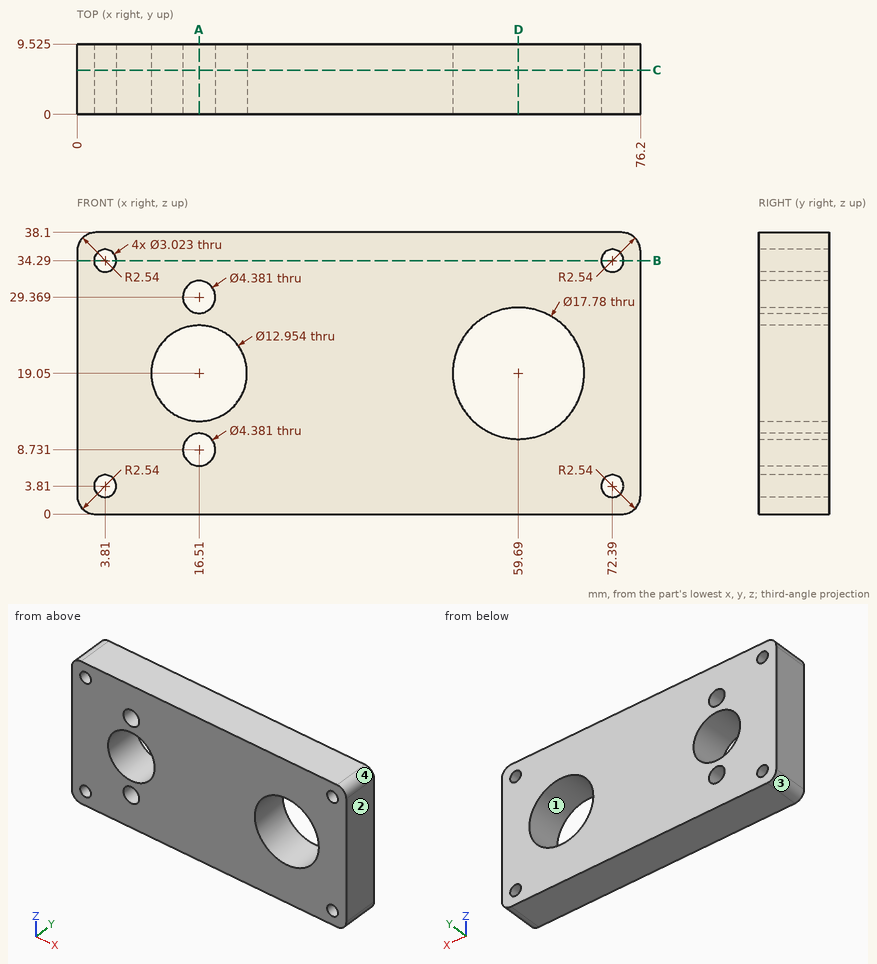
Verification items for this drawing (mm, ordinates from the low corner). Coordinates: 2 decimals unless noted, no trailing zeros. Loops run counter-clockwise (first coordinate to the right, second up) from the corner with the lowest first, then second, coordinate; pieces in that order, holes last. Notation, with made-up numbers: (-33, 28.5) -> (-26, 28.5) arc R18 cw to (-26, 62.5) -> close; hole circle Ø1 at (-21, 62). An arc over 180 degrees is marked (long way). Put each result on its own line as item: value.
1. Section check A-A, the plane x = 16.51. Record the boundary of the cut face in (y, z) (1 decimal), then the cut area to 3 significant figures.
Result set:
outline: (0, 0) -> (9.5, 0) -> (9.5, 6.5) -> (0, 6.5) -> close; (0, 10.9) -> (9.5, 10.9) -> (9.5, 12.6) -> (0, 12.6) -> close; (0, 25.5) -> (9.5, 25.5) -> (9.5, 27.2) -> (0, 27.2) -> close; (0, 31.6) -> (9.5, 31.6) -> (9.5, 38.1) -> (0, 38.1) -> close
area: 156 mm^2
2. Section check D-D, the plane x = 59.69. Record the boundary of the cut face in (y, z) (1 decimal).
Result set:
outline: (0, 0) -> (9.5, 0) -> (9.5, 10.2) -> (0, 10.2) -> close; (0, 27.9) -> (9.5, 27.9) -> (9.5, 38.1) -> (0, 38.1) -> close
3. Section check B-B, the plane z = 34.29. Record the boundary of the cut face in (x, y) (1 decimal).
Result set:
outline: (0, 0) -> (2.3, 0) -> (2.3, 9.5) -> (0, 9.5) -> close; (5.3, 0) -> (70.9, 0) -> (70.9, 9.5) -> (5.3, 9.5) -> close; (73.9, 0) -> (76.2, 0) -> (76.2, 9.5) -> (73.9, 9.5) -> close
4. Gauge pin test, flat ends, axial feed: P1, Ø6, axis at x = 60, z = 27.5, coming from the +Y side (1 decimal); P2, Ø10.5, axis at x = 59.69, z = 19.05, coming from the +Y side. Record the tip position at first contact, or that the pin passes through.
Result set:
P1: stops at y = 9.5
P2: passes through
5. Thickness scan on line 1 (Z direction, x = 3.81, y = 2.25); line 2 (X direction, y = 6, z = 29.5); line 3 (X direction, y = 7.5, z = 23) (1 decimal). Record the ranges inside material, lowest first.
Result set:
line 1: z = 0 to 2.3, 5.32 to 32.78, 35.8 to 38.1
line 2: x = 0 to 14.32, 18.7 to 76.2
line 3: x = 0 to 11.4, 21.6 to 51.7, 67.7 to 76.2
6. Mould release check, pull along Z, two halves, no side actions. Record for the marked faces 1, 2, 3 and 4: pulls with the +Z half, pulls with the -Z half, needs draft (parallel to the pull), parting line crosses it, or undercut.
Result set:
face 1: undercut
face 2: needs draft
face 3: pulls with the -Z half
face 4: pulls with the +Z half
7. Section check C-C, the plane y = 6. Give the number of separate pieces and of enclosed holes in the cut face, then the cut area to 3 significant figures.
Result set:
separate pieces: 1
enclosed holes: 8
area: 2,460 mm^2
